Autodesk Fusion 360 part; units mm, degrees
sketch "Sketch1" plane through (0, 0, 0) normal (0, 1, 0) x (1, 0, 0)
  line L0 (0.4, 76.2) -> (0, 76.2)
  line L1 (12.7, 63.5) -> (12.7, -61.1)
  line L2 (0, -73.8) -> (0.4, -73.8)
  line L3 (-12.3, -61.1) -> (-12.3, 63.5)
  line L4 (-61.1, 12.7) -> (63.5, 12.7)
  line L5 (76.2, 0) -> (76.2, 0.4)
  line L6 (63.5, -12.3) -> (-61.1, -12.3)
  line L7 (-73.8, 0.4) -> (-73.8, 0)
  circle A0 centre (-63.5, 0) radius 4.225
  circle A1 centre (0, 63.5) radius 4.225
  circle A2 centre (63.5, 0) radius 4.225
  circle A3 centre (0, -63.5) radius 4.225
  arc A4 (-73.8, 0.4) -> (-61.1, -12.3) centre (-61.1, 0.4) ccw
  arc A5 (-61.1, 12.7) -> (-73.8, 0) centre (-61.1, 0) ccw
  arc A6 (0.4, 76.2) -> (-12.3, 63.5) centre (0.4, 63.5) ccw
  arc A7 (12.7, 63.5) -> (0, 76.2) centre (0, 63.5) ccw
  arc A8 (76.2, 0) -> (63.5, 12.7) centre (63.5, 0) ccw
  arc A9 (63.5, -12.3) -> (76.2, 0.4) centre (63.5, 0.4) ccw
  arc A10 (-12.3, -61.1) -> (0.4, -73.8) centre (0.4, -61.1) ccw
  arc A11 (0, -73.8) -> (12.7, -61.1) centre (0, -61.1) ccw
  point P0 (-12.3, 76.2)
  point P1 (12.7, 76.2)
  point P2 (-12.3, -73.8)
  point P3 (-73.8, 12.7)
  point P4 (76.2, 12.7)
  point P5 (-73.8, -12.3)
  dimension "d3" = 25
  dimension "d4" = 150
  dimension "d5" = 150
  dimension "d6" = 25
  dimension "d7" = 8.45
  dimension "d8" = 8.45
  dimension "d9" = 8.45
  dimension "d10" = 8.45
  dimension "d11" = 12.7
extrude "Extrude1" add sketch "Sketch1" along normal blind 4
Build history of the part. All positions in model axes, mm. A direction names the side the tool comes from. Round coordinates to 2 decimals unless told otherwise and drop trailing zeros. Write each loop counter-clockwise with the first axis right and the second up, starting at its lowest first coordinate (ties: lowest second). Pieces come first, ordered by that corner, then holes. Notation, with made-up numbers: M 18.25,-10 L 70.25,-10 A21 cw 70.25,28 Z; hole C 57,-28 d8. An arc over 180 degrees is marked long. Answer as a JSON object with one key per item and string values. Group by question number.
(1) Cut at D-D (z = 15). Give the cut face in (x, y), and give its area (3 significant figures).
(2) Cut at A-A (y = 1.9). Give the cut face in (x, z) (3 decimals), and give its area (3 significant figures).
(3) Which spindle directions (+Z, -Z, +X, -X, +Y, -Y) get a long thin tool onto all of the face, cutting with end or side? Do faces 1 (the cylindrical face through (-8.55, 1.97, 70.11)), 2 (the flat face through (12.7, 2, 36)), 3 (the flat face through (12.7, 2, -38)). Say none if no direction does.
(4) Mould opens along Z. For faces 4 (the cylindrical face through (-59.47, 1.97, 1.27)), 5 (the flat face through (38, 2, 12.3)), 6 (the cylindrical face through (67.53, 1.97, 1.27)), 7 (the flat face through (-37, 2, -12.7)) say: pulls with the +Z half, pulls with the -Z half, needs draft (parallel to the pull), parting line crosses it, or undercut.
(5) Drill centre lines: L1, parallel to Z at x = 0, y = 1.1 (3 decimals); L2, parallel to X at y = 2.7, z = 0.5; L3, parallel to Z at x = 63.5, y = 2.9 (3 decimals). Where is each one in solid material? Low to high.
(6) Cut at B-B (x = 65.5). Give the cut face in (y, z), and give its area (3 significant figures).
(7) Cut at C-C (z = 63.5). Give the cut face in (x, y) (3 decimals).
(8) Flat gauge pins, fed straight in: pin 1 (1.5 mm diameter, centred on y = 1, z = 48, fed in from -X); pin 2 (2 mm diameter, centred on y = 2, z = -26, fed in from +X); pin 3 (1.2 mm diameter, centred on x = -29, y = 1, fed in from -Z). Where does each tip first touch, or does it go through?
Responses:
{
 "1": {"outline": "M -12.3,0 L 12.7,0 L 12.7,4 L -12.3,4 Z", "area": "100 mm2"},
 "2": {"outline": "M -73.798,-0.2 A12.7 ccw -61.1,-12.7 L -12.3,-12.7 L -12.3,-63.5 A12.7 ccw 0.2,-76.198 A12.7 ccw 12.7,-63.5 L 12.7,-12.7 L 63.5,-12.7 A12.7 ccw 76.198,-0.2 A12.7 ccw 63.5,12.3 L 12.7,12.3 L 12.7,61.1 A12.7 ccw 0.2,73.798 A12.7 ccw -12.3,61.1 L -12.3,12.3 L -61.1,12.3 A12.7 ccw Z; hole C -63.5,0 d8.45; hole C 0,-63.5 d8.45; hole C 0,63.5 d8.45; hole C 63.5,0 d8.45", "area": "6,370 mm2"},
 "3": {"face 1": "+Z, -X, +Y, -Y", "face 2": "+Z, +X, +Y, -Y", "face 3": "-Z, +X, +Y, -Y"},
 "4": {"face 4": "undercut", "face 5": "pulls with the +Z half", "face 6": "undercut", "face 7": "pulls with the -Z half"},
 "5": {"L1": "z = -76.194 to -67.725, -59.275 to 59.275, 67.725 to 73.794", "L2": "x = -73.77 to -67.7, -59.3 to 59.3, 67.7 to 76.17", "L3": "z = -12.7 to -4.225, 4.225 to 12.3"},
 "6": {"outline": "M 0,-12.54 L 4,-12.54 L 4,-3.72 L 0,-3.72 Z; M 0,3.72 L 4,3.72 L 4,12.14 L 0,12.14 Z", "area": "69.0 mm2"},
 "7": {"outline": "M -12.071,0 L -4.225,0 L -4.225,4 L -12.071,4 Z; M 4.225,0 L 12.471,0 L 12.471,4 L 4.225,4 Z"},
 "8": {"pin 1": "stops at x = -12.3", "pin 2": "stops at x = 12.7", "pin 3": "stops at z = -12.7"}
}
